```python
from build123d import *

# Parameters (mm, degrees)
SKETCH1_R           = 18.5
BOSS_EXTRUDE1_DEPTH = 21
SKETCH2_R           = 16.5
BOSS_EXTRUDE2_DEPTH = 27
SKETCH3_R           = 7
BOSS_EXTRUDE3_DEPTH = 6
BOSS_EXTRUDE4_DEPTH = 3.5
SKETCH5_W           = 40
SKETCH5_H           = 3.5
BOSS_EXTRUDE5_DEPTH = 40
FILLET1_R           = 3
SKETCH6_R           = 6
BOSS_EXTRUDE6_DEPTH = 6
SKETCH7_R           = 3
BOSS_EXTRUDE7_DEPTH = 15
FILLET2_R           = 0.5
CUT_EXTRUDE1_START  = -12
CUT_EXTRUDE1_DEPTH  = 12
CUT_EXTRUDE2_REACH  = 76.33
SKETCH9_R           = 1.5


with BuildPart() as part:
    # Sketch1 → Boss-Extrude1 (new body)
    with BuildSketch(Plane.XY):
        with Locations(Location((0, 0, 0), (0, 0, 180))):
            Circle(SKETCH1_R)
    extrude(amount=BOSS_EXTRUDE1_DEPTH)

    # Sketch2 → Boss-Extrude2 (add)
    with BuildSketch(Plane.XY.offset(21)):
        Circle(SKETCH2_R)
    extrude(amount=BOSS_EXTRUDE2_DEPTH)

    # Sketch3 → Boss-Extrude3 (add)
    with BuildSketch(Plane.XY.offset(48)):
        Circle(SKETCH3_R)
    extrude(amount=BOSS_EXTRUDE3_DEPTH)

    # Sketch4 → Boss-Extrude4 (add)
    with BuildSketch(Plane(origin=(0, 0, 0), x_dir=(-1, 0, 0), z_dir=(0, 0, -1))):
        with BuildLine():
            Line((-20, 0), (-20, -27))
            Line((-20, -27), (20, -27))
            Line((20, -27), (20, 0))
            ThreePointArc((20, 0), (0, 20), (-20, 0))
        make_face()
        with BuildLine():
            Line((6.5, 5), (6.5, -8.5))
            ThreePointArc((6.5, -8.5), (0, -15), (-6.5, -8.5))
            Line((-6.5, -8.5), (-6.5, 5))
            ThreePointArc((-6.5, 5), (0, 11.5), (6.5, 5))
        make_face(mode=Mode.SUBTRACT)
    extrude(amount=BOSS_EXTRUDE4_DEPTH)

    # Sketch5 → Boss-Extrude5 (add)
    with BuildSketch(Plane.XY):
        with Locations((0, -25.25)):
            Rectangle(SKETCH5_W, SKETCH5_H)
    extrude(amount=BOSS_EXTRUDE5_DEPTH)

    # Fillet1
    fillet1_edges = [part.edges().sort_by_distance(p)[0] for p in [
        (0, -27, -3.5),
        (0, -23.5, 0),
        (20, -25.25, 40),
        (-20, -25.25, 40),
    ]]
    fillet(fillet1_edges, radius=FILLET1_R)

    # Sketch6 → Boss-Extrude6 (add)
    with BuildSketch(Plane(origin=(0, 0, 0), x_dir=(-1, 0, 0), z_dir=(0, 0, -1))):
        with Locations(Location((0, -8.5, 0), (0, 0, 180))):
            Circle(SKETCH6_R)
    extrude(amount=BOSS_EXTRUDE6_DEPTH)

    # Sketch7 → Boss-Extrude7 (add)
    with BuildSketch(Plane(origin=(0, 0, -6), x_dir=(-1, 0, 0), z_dir=(0, 0, -1))):
        with Locations((0, -8.5)):
            Circle(SKETCH7_R)
    extrude(amount=BOSS_EXTRUDE7_DEPTH)

    # Fillet2
    fillet2_edges = [part.edges().sort_by_distance(p)[0] for p in [
        (3, -8.5, -21),
    ]]
    fillet(fillet2_edges, radius=FILLET2_R)

    # Sketch8 → Cut-Extrude1 (cut)
    with BuildSketch(Plane(origin=(0, 0, -21), x_dir=(-1, 0, 0), z_dir=(0, 0, -1)).offset(CUT_EXTRUDE1_START)):
        with BuildLine():
            Line((-1.658312395, -6), (1.658312395, -6))
            ThreePointArc((1.658312395, -6), (0, -5.5), (-1.658312395, -6))
        make_face()
    extrude(amount=CUT_EXTRUDE1_DEPTH, mode=Mode.SUBTRACT)

    # Sketch9 → Cut-Extrude2 (cut, up to next)
    with BuildSketch(Plane.XZ.offset(27), mode=Mode.PRIVATE) as cut_extrude2_sk1:
        with Locations(Location((15, 33.5, 0), (0, 0, 270))):
            Circle(SKETCH9_R)
    cut_extrude2_tool1 = extrude(cut_extrude2_sk1.sketch, amount=-CUT_EXTRUDE2_REACH, mode=Mode.PRIVATE) & part.part
    # Sketch9 → Cut-Extrude2 (cut, up to next)
    with BuildSketch(Plane.XZ.offset(27), mode=Mode.PRIVATE) as cut_extrude2_sk2:
        with Locations(Location((15, 9.5, 0), (0, 0, 270))):
            Circle(SKETCH9_R)
    cut_extrude2_tool2 = extrude(cut_extrude2_sk2.sketch, amount=-CUT_EXTRUDE2_REACH, mode=Mode.PRIVATE) & part.part
    # Sketch9 → Cut-Extrude2 (cut, up to next)
    with BuildSketch(Plane.XZ.offset(27), mode=Mode.PRIVATE) as cut_extrude2_sk3:
        with Locations(Location((-15, 33.5, 0), (0, 0, 270))):
            Circle(SKETCH9_R)
    cut_extrude2_tool3 = extrude(cut_extrude2_sk3.sketch, amount=-CUT_EXTRUDE2_REACH, mode=Mode.PRIVATE) & part.part
    # Sketch9 → Cut-Extrude2 (cut, up to next)
    with BuildSketch(Plane.XZ.offset(27), mode=Mode.PRIVATE) as cut_extrude2_sk4:
        with Locations(Location((-15, 9.5, 0), (0, 0, 270))):
            Circle(SKETCH9_R)
    cut_extrude2_tool4 = extrude(cut_extrude2_sk4.sketch, amount=-CUT_EXTRUDE2_REACH, mode=Mode.PRIVATE) & part.part
    add(cut_extrude2_tool1.solids().sort_by_distance((15, -27, 33.5))[0], mode=Mode.SUBTRACT)
    add(cut_extrude2_tool2.solids().sort_by_distance((15, -27, 9.5))[0], mode=Mode.SUBTRACT)
    add(cut_extrude2_tool3.solids().sort_by_distance((-15, -27, 33.5))[0], mode=Mode.SUBTRACT)
    add(cut_extrude2_tool4.solids().sort_by_distance((-15, -27, 9.5))[0], mode=Mode.SUBTRACT)


solid = part.part
```
Work out the finished part from the listing and answer in its coordinate system (mm). A direction names the side the tool comes from. Give positions to 0.01 mm unless a question says otherwise; leave off trailing zeros. Write each loop counter-clockwise with the first axis right and the second up, starting at its lowest first coordinate (ties: lowest second). Pieces come first, ordered by that corner, then holes. Notation, with made-up numbers: (-15, 9) - (13, 9) arc R8 cw to (13, 21) - close; hole circle Ø6 at (47.5, 73.25). An arc over 180 degrees is marked (long way). Use one line per item in the form item = value.
1. Consider L1, parallel to X at y = -24.35, z = 33.5; L2, parallel to X at y = -25, z = 33; L3, parallel to Z at x = -14, y = -13. Determine where each line is inside the solid, lowest interval first.
Filled in:
L1 = -20 to -16.5, -13.5 to 13.5, 16.5 to 20
L2 = -20 to -16.41, -13.59 to 13.59, 16.41 to 20
L3 = -3.5 to 0
2. A cutting plane is placed at C-C (x = 15). Write down the section's boundary in (y, z).
Filled in:
outline = (-27, -0.5) arc R3 ccw to (-24, -3.5) - (13.23, -3.5) - (13.23, 0) - (10.83, 0) - (10.83, 21) - (6.87, 21) - (6.87, 48) - (-6.87, 48) - (-6.87, 21) - (-10.83, 21) - (-10.83, 0) - (-20.5, 0) arc R3 cw to (-23.5, 3) - (-23.5, 8) - (-27, 8) - close; (-27, 11) - (-23.5, 11) - (-23.5, 32) - (-27, 32) - close; (-27, 35) - (-23.5, 35) - (-23.5, 40) - (-27, 40) - close
3. Each of these flat-tipped pins is pushed along its axis until it touches: pin 1 Ø2.5 at (x, z) = (15, 9.5) entering from +Y; pin 2 Ø3.5 at (x, z) = (1, -18) entering from +Y; pin 3 Ø5 at (y, z) = (-18.5, 9) entering from +X; pin 4 Ø5 at (x, z) = (15, 33.5) entering from -Y. Where does it stop, or does it pass through?
Filled in:
pin_1 = 12.38
pin_2 = -6
pin_3 = 9.29
pin_4 = -27
4. For faces 4 (the face through (-3, -7, -6)), 5 (the face through (15.24, -6.32, 34.31)), 6 (the face through (0, -6, -15)), determine the directions among +Z, -Z, +X, -X, +Y, -Y from which every point of the face is accessible in a straight line to the end or side of a thin tool.
Filled in:
face_4 = -Z
face_5 = +Z
face_6 = -Z, +X, -X, +Y
5. A cutting plane is placed at D-D (y = -3.5). Write down the section's boundary in (x, z).
Filled in:
outline = (-20, -3.5) - (-6.5, -3.5) - (-6.5, 0) - (-3.32, 0) - (-3.32, -6) - (3.32, -6) - (3.32, 0) - (6.5, 0) - (6.5, -3.5) - (20, -3.5) - (20, 0) - (18.17, 0) - (18.17, 21) - (16.12, 21) - (16.12, 48) - (6.06, 48) - (6.06, 54) - (-6.06, 54) - (-6.06, 48) - (-16.12, 48) - (-16.12, 21) - (-18.17, 21) - (-18.17, 0) - (-20, 0) - close
6. Determine the mould class of faces 1 (the face through (0.28, -22.6, 0.86)), 2 (the face through (-20, -24, 12)), 3 (the face through (-15, -25, 11)) for opening direction Z: released by +Z, released by -Z, zero draft, split by the parting line, or undercut.
Filled in:
face_1 = released by +Z
face_2 = zero draft
face_3 = undercut
7. A cutting plane is placed at B-B (z = 30). Write down the section's boundary in (x, y).
Filled in:
outline = (-20, -27) - (20, -27) - (20, -23.5) - (-20, -23.5) - close; circle Ø33 at (0, 0)
8. A cutting plane is placed at A-A (z = -2). Write down the section's boundary in (x, y).
Filled in:
outline = (-20, -26.6) - (20, -26.6) - (20, 0) arc R20 ccw to (-20, 0) - close; circle Ø12 at (0, -8.5); hole (-6.5, -8.5) arc R6.5 ccw to (6.5, -8.5) - (6.5, 5) arc R6.5 ccw to (-6.5, 5) - close
